from build123d import *

# Parameters (mm, degrees)
SKETCH1_R           = 1.975
BOSS_EXTRUDE1_DEPTH = 4.5


with BuildPart() as part:
    # Sketch1 → Boss-Extrude1 (new body)
    with BuildSketch(Plane(origin=(0, 0, 0), x_dir=(1, 0, 0), z_dir=(0, 1, 0))):
        with BuildLine():
            Line((65, 20.3), (19.8, 20.3))
            Line((19.8, 20.3), (19.8, 11.37))
            Line((19.8, 11.37), (10.87, 11.37))
            Line((10.87, 11.37), (10.87, 18.3))
            ThreePointArc((10.87, 18.3), (10.284213562, 19.714213562), (8.87, 20.3))
            Line((8.87, 20.3), (-65, 20.3))
            Line((-65, 20.3), (-65, -20.3))
            Line((-65, -20.3), (65, -20.3))
            Line((65, -20.3), (65, 20.3))
        make_face()
        with Locations(Location((-61.05, 16.35, 0), (0, 0, 270))):
            Circle(SKETCH1_R, mode=Mode.SUBTRACT)
        with Locations(Location((61.05, 16.35, 0), (0, 0, 90))):
            Circle(SKETCH1_R, mode=Mode.SUBTRACT)
        with Locations(Location((61.05, -16.35, 0), (0, 0, 270))):
            Circle(SKETCH1_R, mode=Mode.SUBTRACT)
        with Locations(Location((-61.05, -16.35, 0), (0, 0, 90))):
            Circle(SKETCH1_R, mode=Mode.SUBTRACT)
        with Locations(Location((-25.55, 16.35, 0), (0, 0, 270))):
            Circle(SKETCH1_R, mode=Mode.SUBTRACT)
        with Locations(Location((-5.328324842, -2.339651524, 0), (0, 0, 270))):
            Circle(SKETCH1_R, mode=Mode.SUBTRACT)
    extrude(amount=BOSS_EXTRUDE1_DEPTH)


solid = part.part
Build history of the part. All positions in model axes, mm. A direction names the side the tool comes from. Round coordinates to 2 decimals unless told otherwise and drop trailing zeros. Write each loop counter-clockwise with the first axis right and the second up, starting at its lowest first coordinate (ties: lowest second). Pieces come first, ordered by that corner, then holes. Notation, with made-up numbers: M -38,-7.75 L -16,-7.75 A24 cw -16,3.25 Z; hole C 21.25,58 d8. An arc over 180 degrees is marked long. Answer as a JSON object with one key per item and string values. Group by question number.
(1) Cut at A-A (z = -16.35). Give the cut face in (x, y) (3 decimals).
(2) Cut at B-B (x = 61.05). Give the cut face in (y, z) (3 decimals), and give its area (3 significant figures).
(3) Which spindle directions (+Z, -Z, +X, -X, +Y, -Y) get a long thin tool onto all of the face, cutting with end or side? Do faces 5 (the flat face through (15, 2, -11.37)), 6 (the cylindrical face through (61.643, 2.218, 18.234)). Say none if no direction does.
(4) Drill centre lines: L1, parallel to X at y = 3.55, z = 16.5; L2, parallel to X at y = 2.35, z = -16.35 (3 decimals); L3, parallel to X at y = 2.9, z = 15. Where is each one in solid material? Low to high.
(5) Mould opens along Z. For faces 1 (the cylindrical face through (-3.66, 2.22, 3.4)), 2 (the flat face through (-1, 2, 20.3)), 3 (the flat face through (-28, 2, -20.3)), 4 (the flat face through (-1, 4.5, 0)) say: pulls with the +Z half, pulls with the -Z half, needs draft (parallel to the pull), parting line crosses it, or undercut.
(6) Cut at C-C (z = 1.5). Give the cut face in (x, y).
(7) Cut at D-D (y = 3.2). Give the cut face in (x, z) (3 decimals), and give its area (3 significant figures).
Responses:
{
 "1": {"outline": "M -65,0 L -63.025,0 L -63.025,4.5 L -65,4.5 Z; M -59.075,0 L -27.525,0 L -27.525,4.5 L -59.075,4.5 Z; M -23.575,0 L 10.87,0 L 10.87,4.5 L -23.575,4.5 Z; M 19.8,0 L 59.075,0 L 59.075,4.5 L 19.8,4.5 Z; M 63.025,0 L 65,0 L 65,4.5 L 63.025,4.5 Z"},
 "2": {"outline": "M 0,-20.3 L 4.5,-20.3 L 4.5,-18.325 L 0,-18.325 Z; M 0,-14.375 L 4.5,-14.375 L 4.5,14.375 L 0,14.375 Z; M 0,18.325 L 4.5,18.325 L 4.5,20.3 L 0,20.3 Z", "area": "147 mm2"},
 "3": {"face 5": "-Z, +Y, -Y", "face 6": "+Y, -Y"},
 "4": {"L1": "x = -65 to -63.02, -59.08 to 59.08, 63.02 to 65", "L2": "x = -65 to -63.025, -59.075 to -27.525, -23.575 to 10.87, 19.8 to 59.075, 63.025 to 65", "L3": "x = -65 to -62.49, -59.61 to 59.61, 62.49 to 65"},
 "5": {"face 1": "undercut", "face 2": "pulls with the +Z half", "face 3": "pulls with the -Z half", "face 4": "needs draft"},
 "6": {"outline": "M -65,0 L -7.12,0 L -7.12,4.5 L -65,4.5 Z; M -3.54,0 L 65,0 L 65,4.5 L -3.54,4.5 Z"},
 "7": {"outline": "M -65,-20.3 L 8.87,-20.3 A2 ccw 10.87,-18.3 L 10.87,-11.37 L 19.8,-11.37 L 19.8,-20.3 L 65,-20.3 L 65,20.3 L -65,20.3 Z; hole C -61.05,-16.35 d3.95; hole C -61.05,16.35 d3.95; hole C -25.55,-16.35 d3.95; hole C -5.328,2.34 d3.95; hole C 61.05,-16.35 d3.95; hole C 61.05,16.35 d3.95", "area": "5,120 mm2"}
}
